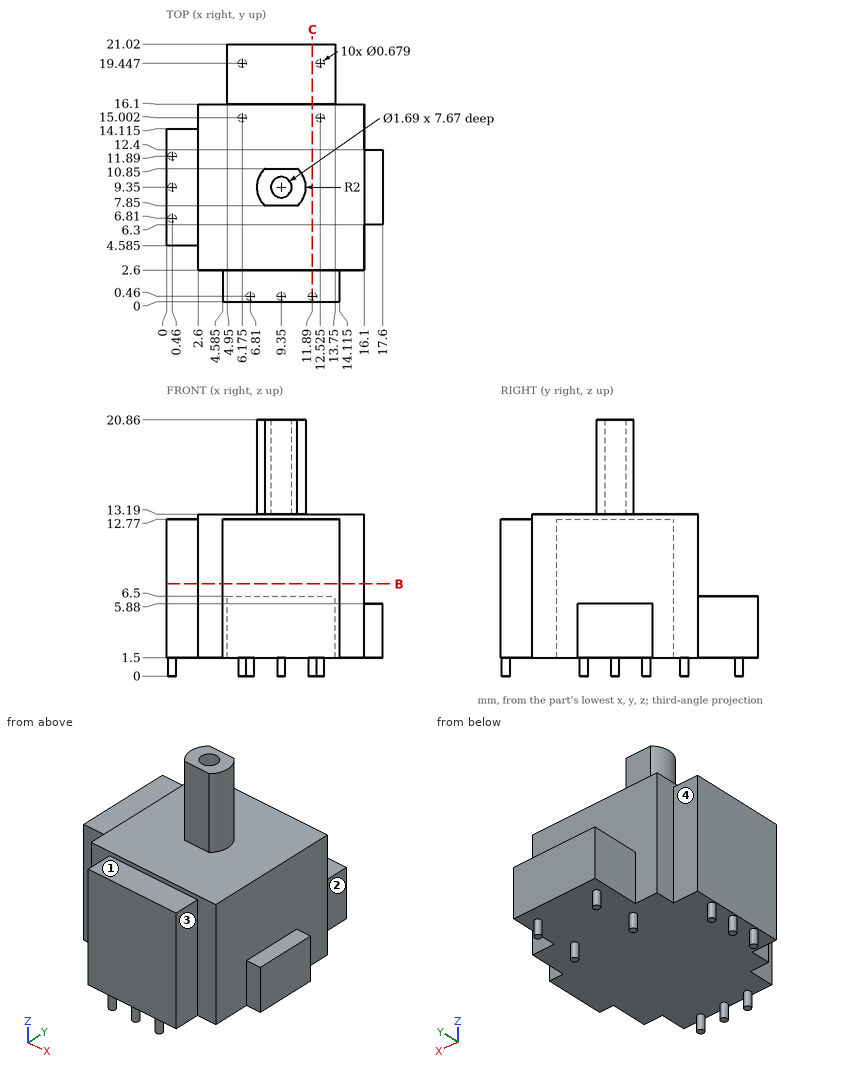
The figure shows three views and two pictorial views of one solid part (mm, origin at its lowest corner). Answer the questions. A direction names the side the tool comes from. Round coordinates to 2 decimals unless told otherwise and drop trailing zeros. Order: outer loops, then holes, each group sorted by start corner. A loop starts at its lowest first (then second) coordinate and runs counter-clockwise, first axis right, second up. Notation, with made-up numbers: M 68,-4 L 108,-4 A16 cw 108,10 Z; hole C -7.5,20.5 d6. An arc over 180 degrees is marked long. Answer in a Markdown table with one row per item. Add a question column.
1) Flat-ended cylindrical pins translate along their axes: pin 1 Ø8 at (y, z) = (6.5, 10.5) entering from +X; pin 2 Ø6 at (x, z) = (8.5, 7.5) entering from +Y; pin 3 Ø1.6 at (x, y) = (17, 10) entering from +Z; pin 4 Ø10 at (x, z) = (13, 12.5) entering from +Y. Find the tip coordinate at first contact, or state that the pin passes through.
2) Which of the six approach directions +Z, -Z, +X, -X, +Y, -Y give full straight-line access (tool end or side, diameter ignored) to the marked faces 1, 2, 3 and 4?
3) The part is cut by section C-C on x = 11.89. Determine the outline of the cut face in (y, z), plus the area to 3 significant figures.
4) The part is cut by section B-B on z = 7.5. Determine the outline of the cut face in (x, y) (1 decimal), plus the area to 3 significant figures.
5) Consider line 1 along Z through (x, y) = (7.25, 1); line 2 along Z through (x, y) = (7.25, 16.5); line 3 along X through (y, z) = (5.75, 13). Determine where each line is inside the solid, lowest interval first. Write a range as from..to.
Findings below:
| question | item | result |
|---|---|---|
| 1 | pin 1 | stops at x = 16.1 |
| 1 | pin 2 | stops at y = 21.02 |
| 1 | pin 3 | stops at z = 5.88 |
| 1 | pin 4 | stops at y = 16.1 |
| 2 | face 1 | +Z, +X, -X, -Y |
| 2 | face 2 | +Z, -Z, +X, +Y |
| 2 | face 3 | +Z, -Z, +X, -Y |
| 2 | face 4 | +Z, -Z, -X, +Y |
| 3 | outline | M 0,1.5 L 0.12,1.5 L 0.12,0 L 0.8,0 L 0.8,1.5 L 21.02,1.5 L 21.02,6.5 L 16.1,6.5 L 16.1,13.19 L 2.6,13.19 L 2.6,12.77 L 0,12.77 Z |
| 3 | area | 213 mm² |
| 4 | outline | M 0,4.6 L 2.6,4.6 L 2.6,2.6 L 4.6,2.6 L 4.6,0 L 14.1,0 L 14.1,2.6 L 16.1,2.6 L 16.1,16.1 L 2.6,16.1 L 2.6,14.1 L 0,14.1 Z |
| 4 | area | 232 mm² |
| 5 | line 1 | z = 1.5..12.77 |
| 5 | line 2 | z = 1.5..6.5 |
| 5 | line 3 | x = 2.6..16.1 |
